```python
from build123d import *

# Parameters (mm, degrees)
SKETCH1_R           = 0.5
BOSS_EXTRUDE1_DEPTH = 0.5


with BuildPart() as part:
    # Sketch1 → Boss-Extrude1 (new body)
    with BuildSketch(Plane(origin=(0, 0, 0), x_dir=(1, 0, 0), z_dir=(0, 1, 0))):
        with BuildLine():
            Line((9.965, 2.9), (14.065, 2.9))
            ThreePointArc((14.065, 2.9), (14.418553391, 2.753553391), (14.565, 2.4))
            Line((14.565, 2.4), (14.565, -2.4))
            ThreePointArc((14.565, -2.4), (14.418553391, -2.753553391), (14.065, -2.9))
            Line((14.065, -2.9), (-6.445, -2.9))
            ThreePointArc((-6.445, -2.9), (-6.798553391, -2.753553391), (-6.945, -2.4))
            Line((-6.945, -2.4), (-6.945, 2.4))
            ThreePointArc((-6.945, 2.4), (-6.798553391, 2.753553391), (-6.445, 2.9))
            Line((-6.445, 2.9), (-2.345, 2.9))
            Line((-2.345, 2.9), (-2.345, 4.1))
            Line((-2.345, 4.1), (9.965, 4.1))
            Line((9.965, 4.1), (9.965, 2.9))
        make_face()
        with Locations(Location((0, 0, 0), (0, 0, 270))):
            Circle(SKETCH1_R, mode=Mode.SUBTRACT)
        with Locations(Location((3.81, 0, 0), (0, 0, 270))):
            Circle(SKETCH1_R, mode=Mode.SUBTRACT)
        with Locations(Location((7.62, 0, 0), (0, 0, 270))):
            Circle(SKETCH1_R, mode=Mode.SUBTRACT)
    extrude(amount=BOSS_EXTRUDE1_DEPTH)


solid = part.part
```
Model file for the job. Use its own axes, mm. Give positions to 0.01 mm unless a question says otherwise; leave off trailing zeros. Loops run counter-clockwise (first coordinate to the right, second up) from the corner with the lowest first, then second, coordinate; pieces in that order, holes last. Notation, with made-up numbers: (-13, 46.5) -> (-7, 46.5) arc R22 ccw to (-7, 76.5) -> close; hole circle Ø11 at (-16, 15.5). An arc over 180 degrees is marked (long way). Use CSV: the item, a comma, the result in double quotes. Start each with the question number.
1) Slice it at D-D on x = -3.75. Give the cut face in (y, z).
2) Slice it at B-B on x = 3.81. Give the cut face in (y, z), plus the area to 3 significant figures.
3) Slice it at C-C on y = 0.35. Give the cut face in (x, z) (3 decimals), plus the area to 3 significant figures.
4) Slice it at A-A on z = 0. Give the cut face in (x, y) (3 decimals).
5) Wall check: line 1 (X direction, y = 0.4, z = 0) (3 decimals); line 2 (Z direction, x = 13.25, y = 0.45); line 3 (Z direction, x = 4.25, y = 0.3). Give the ranges that are in metal, low to high.
6) Mould opens along Z. For faces 1 (the flat face through (4, 0.5, -1)), 2 (the cylindrical face through (4.3, 0.2, -0.1)) say: released by +Z, released by -Z, zero draft, split by the parting line, or undercut.
Computed values:
1,outline,"(0, -2.9) -> (0.5, -2.9) -> (0.5, 2.9) -> (0, 2.9) -> close"
2,outline,"(0, -4.1) -> (0.5, -4.1) -> (0.5, -0.5) -> (0, -0.5) -> close; (0, 0.5) -> (0.5, 0.5) -> (0.5, 2.9) -> (0, 2.9) -> close"
2,area,"3.00 mm^2"
3,outline,"(-6.945, -2.4) arc R0.5 ccw to (-6.445, -2.9) -> (-2.345, -2.9) -> (-2.345, -4.1) -> (9.965, -4.1) -> (9.965, -2.9) -> (14.065, -2.9) arc R0.5 ccw to (14.565, -2.4) -> (14.565, 2.4) arc R0.5 ccw to (14.065, 2.9) -> (-6.445, 2.9) arc R0.5 ccw to (-6.945, 2.4) -> close; hole circle Ø1 at (0, 0); hole circle Ø1 at (3.81, 0); hole circle Ø1 at (7.62, 0)"
3,area,"137 mm^2"
4,outline,"(-6.945, 0) -> (-0.5, 0) -> (-0.5, 0.5) -> (-6.945, 0.5) -> close; (0.5, 0) -> (3.31, 0) -> (3.31, 0.5) -> (0.5, 0.5) -> close; (4.31, 0) -> (7.12, 0) -> (7.12, 0.5) -> (4.31, 0.5) -> close; (8.12, 0) -> (14.565, 0) -> (14.565, 0.5) -> (8.12, 0.5) -> close"
5,line 1,"x = -6.945 to -0.5, 0.5 to 3.31, 4.31 to 7.12, 8.12 to 14.565"
5,line 2,"z = -2.9 to 2.9"
5,line 3,"z = -4.1 to -0.24, 0.24 to 2.9"
6,face 1,"zero draft"
6,face 2,"undercut"
